The listing builds one solid part. Answer for the finished solid, in the listing's coordinates (mm). A direction names the side the tool comes from. Round coordinates to 2 decimals unless told otherwise and drop trailing zeros. Loops run counter-clockwise (first coordinate to the right, second up) from the corner with the lowest first, then second, coordinate; pieces in that order, holes last. Notation, with made-up numbers: (60, 84) -> (113, 84) arc R20 ccw to (113, 88) -> close; hole circle Ø8 at (40, -6). An arc over 180 degrees is marked (long way). Answer in a Markdown table with one row per item. Add a question column.
```python
from build123d import *

# Parameters (mm, degrees)
SKETCH1_W                  = 68.7568
SKETCH1_H                  = 32.004
SKETCH2_R                  = 31.877
BOSS_EXTRUDE1_DEPTH        = 8.2296
SKETCH3_R                  = 15.0368
BOSS_EXTRUDE2_DEPTH        = 5
SKETCH4_R                  = 31.877
BOSS_EXTRUDE3_DEPTH        = 8.2296
SKETCH5_R                  = 9.525
BOSS_EXTRUDE4_DEPTH        = 4
SKETCH6_R                  = 4
BOSS_EXTRUDE5_DEPTH        = 31.6
CUT_EXTRUDE1_REACH         = 31.204
M3_5_CLEARANCE_HOLE1_D     = 4.0386
M3_5_CLEARANCE_HOLE1_DEPTH = 13.6144
M3_5_CLEARANCE_HOLE1_TIP   = 1.213317848
CHAMFER1_SIZE              = 1.016
CHAMFER2_SIZE              = 0.5
FILLET1_R                  = 1


with BuildPart() as part:
    # Sketch1 → Revolve1 (revolve)
    with BuildSketch(Plane.XY):
        with Locations((42.608, 16.002)):
            Rectangle(SKETCH1_W, SKETCH1_H)
    revolve(axis=Axis((8.2296, 0, 0), (1, 0, 0)))

    # Sketch2 → Boss-Extrude1 (add)
    with BuildSketch(Plane(origin=(76.9864, 0, 0), x_dir=(0, 0, -1), z_dir=(1, 0, 0))):
        Circle(SKETCH2_R)
    extrude(amount=BOSS_EXTRUDE1_DEPTH)

    # Sketch3 → Boss-Extrude2 (add)
    with BuildSketch(Plane(origin=(85.216, 0, 0), x_dir=(0, 0, -1), z_dir=(1, 0, 0))):
        Circle(SKETCH3_R)
    extrude(amount=BOSS_EXTRUDE2_DEPTH)

    # Sketch4 → Boss-Extrude3 (add)
    with BuildSketch(Plane.ZY.offset(-8.2296)):
        Circle(SKETCH4_R)
    extrude(amount=BOSS_EXTRUDE3_DEPTH)

    # Sketch5 → Boss-Extrude4 (add)
    with BuildSketch(Plane.ZY):
        Circle(SKETCH5_R)
    extrude(amount=BOSS_EXTRUDE4_DEPTH)

    # Sketch6 → Boss-Extrude5 (add)
    with BuildSketch(Plane.ZY.offset(4)):
        Circle(SKETCH6_R)
    extrude(amount=BOSS_EXTRUDE5_DEPTH)

    # Sketch7 → Cut-Extrude1 (cut, up to next)
    with BuildSketch(Plane.XZ.offset(-2.8), mode=Mode.PRIVATE) as cut_extrude1_sk1:
        with BuildLine():
            Line((-7.1, 1), (-26.6, 1))
            ThreePointArc((-26.6, 1), (-27.6, 0), (-26.6, -1))
            Line((-26.6, -1), (-7.1, -1))
            ThreePointArc((-7.1, -1), (-6.1, 0), (-7.1, 1))
        make_face()
    cut_extrude1_tool1 = extrude(cut_extrude1_sk1.sketch, amount=-CUT_EXTRUDE1_REACH, mode=Mode.PRIVATE) & part.part
    add(cut_extrude1_tool1.solids().sort_by_distance((-16.85, 2.8, 0))[0], mode=Mode.SUBTRACT)

    # Sketch8 → Revolve2 (revolve)
    with BuildSketch(Plane.XY.offset(-18.607090683)):
        Polygon((85.216, 15.525359639), (85.216, 11.207359639), (87.4639, 11.207359639), (87.4639, 13.325359639), (85.2639, 15.525359639), align=None)
    revolve(axis=Axis((85.216, 11.207359639, -18.607090683), (1, 0, 0)))

    # Sketch9 → Revolve3 (revolve)
    with BuildSketch(Plane.XY.offset(-11.207359639)):
        Polygon((85.216, 22.925090683), (85.216, 18.607090683), (87.4639, 18.607090683), (87.4639, 20.725090683), (85.2639, 22.925090683), align=None)
    revolve(axis=Axis((85.216, 18.607090683, -11.207359639), (1, 0, 0)))

    # M3.5 Clearance Hole1
    with Locations(Plane.ZY):
        with Locations((0, 25.4), (0, -25.4)):
            Hole(M3_5_CLEARANCE_HOLE1_D / 2, depth=M3_5_CLEARANCE_HOLE1_DEPTH)
            with Locations((0, 0, -(M3_5_CLEARANCE_HOLE1_DEPTH + M3_5_CLEARANCE_HOLE1_TIP / 2))):  # 118° drill point
                Cone(0, M3_5_CLEARANCE_HOLE1_D / 2, M3_5_CLEARANCE_HOLE1_TIP, mode=Mode.SUBTRACT)

    # Chamfer1
    chamfer1_edges = [part.edges().sort_by_distance(p)[0] for p in [
        (90.216, 0, 15.0368),
        (-4, 0, -9.525),
    ]]
    chamfer(chamfer1_edges, length=CHAMFER1_SIZE)

    # Chamfer2
    chamfer2_edges = [part.edges().sort_by_distance(p)[0] for p in [
        (-35.6, 0, -4),
    ]]
    chamfer(chamfer2_edges, length=CHAMFER2_SIZE)

    # Fillet1
    fillet1_edges = [part.edges().sort_by_distance(p)[0] for p in [
        (0, 0, -31.877),
        (85.216, 0, 31.877),
    ]]
    fillet(fillet1_edges, radius=FILLET1_R)


solid = part.part
```
Item 1: Section C-C, the plane x = 60.5 is taken. Write down the section's boundary in (y, z).
Item 2: Section B-B, the plane x = -10.5 is taken. Write down the section's boundary in (y, z).
Item 3: Consider L1, parallel to Y at x = 3.75, z = 0; L2, parallel to X at y = -15.5, z = -22; L3, parallel to Z at x = 4.5, y = -25.4. Determine where each line is inside the solid, lowest interval first. Write a range as from..to.
Item 4: Flat-ended cylindrical pins translate along their axes: P1, Ø8, axis at x = 14.5, z = 24.5, coming from the -Y side; P2, Ø5.5, axis at y = 25.4, z = 0, coming from the -X side; P3, Ø1.2, axis at x = -19.5, y = 3.5, coming from the -Z side (3 decimals). Find the tip coordinate at first contact, or state that the pin passes through.
Item 5: The mould has two halves that part along Y. Classify faces 1 (the flat face through (-35.6, 0, 0)), 2 (the cylindrical face through (4.665, 9.575, 30.405)), 3 (the cylindrical face through (6.9, -27.37, 0.44)): +Y half, -Y half, draft (parallel to the pull), parting line (faces both ways), or undercut.
Item 6: For faces 4 (the flat face through (87.464, 11, -19)), 5 (the cylindrical face through (80.551, 9.575, -30.405)), 6 (the flat face through (-4, -2, 4)), determine the directions among +Z, -Z, +X, -X, +Y, -Y from which every point of the face is accessible in a straight line to the end or side of a thin tool.
Here are the results:
| question | item | result |
|---|---|---|
| 1 | outline | circle Ø64.01 at (0, 0) |
| 2 | outline | (2.8, -1) -> (2.8, 1) -> (3.87, 1) arc R4 ccw (long way) to (3.87, -1) -> close |
| 3 | L1 | y = -31.88..-27.42, -23.38..23.38, 27.42..31.88 |
| 3 | L2 | x = 0..85.22 |
| 3 | L3 | z = -19.26..-2.02, 2.02..19.26 |
| 4 | P1 | stops at y = -24.58 |
| 4 | P2 | stops at x = 0 |
| 4 | P3 | stops at z = -2.755 |
| 5 | face 1 | draft |
| 5 | face 2 | parting line |
| 5 | face 3 | undercut |
| 6 | face 4 | -Z, +X, +Y, -Y |
| 6 | face 5 | +X |
| 6 | face 6 | -X |
